Check sheet for the drawn part. Datum: minimum x, y, z corner. Units: mm. A direction names the side the tool comes from. Give positions to 0.01 mm unless a question says otherwise; leave off trailing zeros. Order: outer loops, then holes, each group sorted by start corner. A loop starts at its lowest first (then second) coordinate and runs counter-clockwise, first axis right, second up. Notation, with made-up numbers: M 86,46.25 L 131,46.25 A5 ccw 131,53.25 Z; hole C -23,-37.75 d6. An arc over 180 degrees is marked long. Answer in a Markdown table with one row per item. Add a question column.
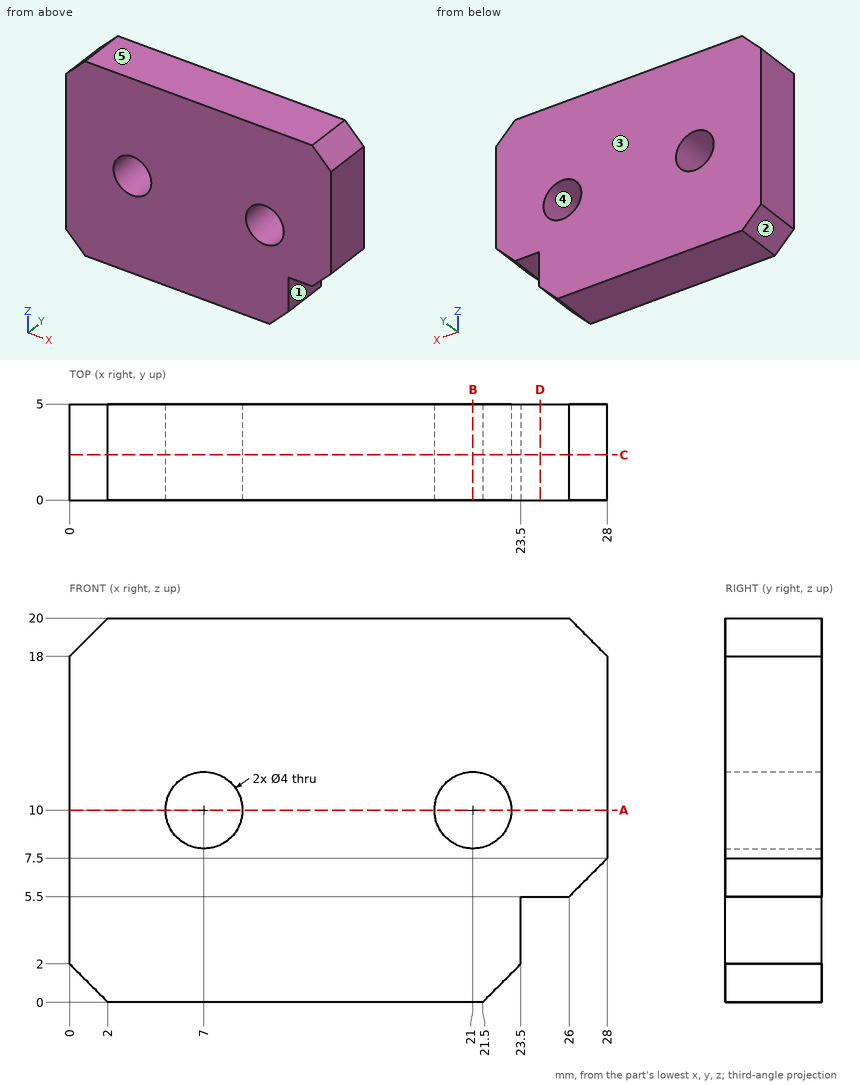
Q1. Cross-section at B-B (x = 21). Record the boundary of the cut face in (y, z).
Q2. Cross-section at D-D (x = 24.5). Record the boundary of the cut face in (y, z), and give its area (3 significant figures).
Q3. Cross-section at A-A (z = 10). Record the boundary of the cut face in (x, y).
Q4. Go/stop test with flat-tipped pins: pin 1 (3 mm diameter, centred on x = 24.5, y = 3, fed in from -Z); pin 2 (2 mm diameter, centred on x = 23, z = 7, fed in from -Y). Record where each tip stops, or that it passes through.
Q5. Tool access check on the marked faces 1 and 2. Record the directions out of +Z, -Z, +X, -X, +Y, -Y that give a thin tool (end or side, any length) a straight path to the whole face; none if there is none.
Q6. Cross-section at C-C (y = 2.35). Record the boundary of the cut face in (x, z).
Q7. Thickness scan on probe 1 along X at (y, z) = (2.15, 10); probe 2 along Z at (x, y) = (7, 1.55); probe 3 along X at (y, z) = (2.55, 8.5). Record the ranges inside material, lowest first.
Q8. Draft check along Z on the marked faces 3, 4 and 5. Enter one of: pulls with the +Z half, pulls with the -Z half, needs draft (parallel to the pull), parting line crosses it, or undercut.
Values follow:
| question | item | result |
|---|---|---|
| 1 | outline | M 0,0 L 5,0 L 5,8 L 0,8 Z; M 0,12 L 5,12 L 5,20 L 0,20 Z |
| 2 | outline | M 0,5.5 L 5,5.5 L 5,20 L 0,20 Z |
| 2 | area | 72.5 mm² |
| 3 | outline | M 0,0 L 5,0 L 5,5 L 0,5 Z; M 9,0 L 19,0 L 19,5 L 9,5 Z; M 23,0 L 28,0 L 28,5 L 23,5 Z |
| 4 | pin 1 | z = 1.5 |
| 4 | pin 2 | y = 0 |
| 5 | face 1 | -Z, +X, +Y, -Y |
| 5 | face 2 | -Z, -X, +Y, -Y |
| 6 | outline | M 0,2 L 2,0 L 21.5,0 L 23.5,2 L 23.5,5.5 L 26,5.5 L 28,7.5 L 28,18 L 26,20 L 2,20 L 0,18 Z; hole C 7,10 d4; hole C 21,10 d4 |
| 7 | probe 1 | 0 to 5, 9 to 19, 23 to 28 |
| 7 | probe 2 | 0 to 8, 12 to 20 |
| 7 | probe 3 | 0 to 5.68, 8.32 to 19.68, 22.32 to 28 |
| 8 | face 3 | needs draft |
| 8 | face 4 | undercut |
| 8 | face 5 | pulls with the +Z half |
